The listing builds one solid part. Answer for the finished solid, in the listing's coordinates (mm). A direction names the side the tool comes from. Round coordinates to 2 decimals unless told otherwise and drop trailing zeros. Loops run counter-clockwise (first coordinate to the right, second up) from the corner with the lowest first, then second, coordinate; pieces in that order, holes last. Notation, with made-up numbers: (-15, 51) -> (-6, 51) arc R20 cw to (-6, 85) -> close; hole circle Ø6 at (53, 30.25). An arc over 180 degrees is marked (long way). One line per question, with ' | ' between items.
from build123d import *

# Parameters (mm, degrees)
F0_W        = 17.78
F0_H        = 8.255
F1_DEPTH    = 2.54
F2_W        = 14.732
F2_H        = 8.128
F3_DEPTH    = 10.16
F4_T1_DEPTH = 40.132


# Not quite as in the source:
# - a fillet or chamfer that OpenCascade refuses, or shapes differently, is made with other operations: its cross-section is extruded or revolved along the edge and cut away or added


with BuildPart() as f1:
    # F0 (on Front) → F1 (new body)
    with BuildSketch(Plane.XZ):
        Rectangle(F0_W, F0_H)
    extrude(amount=F1_DEPTH)

    # F2 (on Front) → F3 (join)
    with BuildSketch(Plane.XZ):
        Rectangle(F2_W, F2_H)
    extrude(amount=F3_DEPTH)

    # F4: fillet of radius 5.08 on 2 edges, made by hand

    # F4_s2 → F4_t1 (cut)
    with BuildSketch(Plane.YZ.offset(-20.066)):
        with BuildLine():
            ThreePointArc((-5.08, 4.064), (-8.6721024484, 2.5761024484), (-10.16, -1.016))
            Line((-10.16, -1.016), (-10.16, 4.064))
            Line((-10.16, 4.064), (-5.08, 4.064))
        make_face()
        with BuildLine():
            ThreePointArc((-5.08, -4.064), (-8.6721024484, -2.5761024484), (-10.16, 1.016))
            Line((-10.16, 1.016), (-10.16, -4.064))
            Line((-10.16, -4.064), (-5.08, -4.064))
        make_face()
    extrude(amount=F4_T1_DEPTH, mode=Mode.SUBTRACT)


solid = f1.part
Q1. A cutting plane is placed at D-D on z = -0.5. Give the vertices of the cut face in (x, y), plus the area to 3 significant figures.
Numbers:
outline: (-8.89, -2.54) -> (-7.37, -2.54) -> (-7.37, -9.93) -> (7.37, -9.93) -> (7.37, -2.54) -> (8.89, -2.54) -> (8.89, 0) -> (-8.89, 0) -> close | area: 154 mm^2
Q2. Find the intervals of material crossed by line 1 (X direction, y = -8, z = -1.5); line 2 (Z direction, x = -3.25, y = -4.75); line 3 (Y direction, x = 1.75, z = 1.75), in increasing order. Write a range as from..to.
Numbers:
line 1: -7.37..7.37 | line 2: -4.06..4.06 | line 3: -9.34..0
Q3. A cutting plane is placed at B-B on x = 5. Give the vertices of the cut face in (y, z), plus the area to 3 significant figures.
Numbers:
outline: (-10.06, 0) arc R5.08 ccw to (-5.08, -4.06) -> (-2.54, -4.06) -> (-2.54, -4.13) -> (0, -4.13) -> (0, 4.13) -> (-2.54, 4.13) -> (-2.54, 4.06) -> (-5.08, 4.06) arc R5.08 ccw to start | area: 71.9 mm^2
Q4. A cutting plane is placed at C-C on y = -6. Give the vertices of the cut face in (x, z), plus the area to 3 significant figures.
Numbers:
outline: (-7.37, -3.98) -> (7.37, -3.98) -> (7.37, 3.98) -> (-7.37, 3.98) -> close | area: 117 mm^2
Q5. Given pin 1 Ø4 at (y, z) = (-7.5, -1.5) entering from -X; pin 2 Ø5 at (x, y) = (0, -7.5) entering from +Z; pin 3 Ø0.8 at (x, y) = (1, -3.5) entering from -Z, each flat-ended and moving along its own axis, determine where each tip first touches the part or whether it passes through.
Numbers:
pin 1: x = -7.37 | pin 2: z = 4.06 | pin 3: z = -4.06
Q6. For faces 1 (the face through (-7.366, -5, 0)), 2 (the face through (0, -4, 4.064)), 3 (the face through (-8.89, -1, 0)), 4 (the face through (7.366, -5, 0)), 5 (the face through (0, -4, -4.064)), determine the directions among +Z, -Z, +X, -X, +Y, -Y from which every point of the face is accessible in a straight line to the end or side of a thin tool.
Numbers:
face 1: +Z, -Z, -X, -Y | face 2: +Z, +X, -X, -Y | face 3: +Z, -Z, -X, +Y, -Y | face 4: +Z, -Z, +X, -Y | face 5: -Z, +X, -X, -Y
Q7. A cutting plane is placed at A-A on z = 2. Give the vertices of the cut face in (x, y).
Numbers:
outline: (-8.89, -2.54) -> (-7.37, -2.54) -> (-7.37, -9.17) -> (7.37, -9.17) -> (7.37, -2.54) -> (8.89, -2.54) -> (8.89, 0) -> (-8.89, 0) -> close
